Part model, mm, in its own coordinate system. Coordinates: 2 decimals unless noted, no trailing zeros.
1) Pin check, flat tips, straight feed: pin 1 Ø1.5 at (x, y) = (-3, 7.5) entering from -Z; pin 2 Ø2.5 at (x, z) = (0.5, -60) entering from +Y; pin 3 Ø1 at (y, z) = (-3, 109) entering from +X; pin 4 Ø1.6 at (y, z) = (0.5, -57.5) entering from -X. Stop position of each tip, or through.
2) Mould opens along Y. For faces 1 (the flat face through (3, 0, 152.4)), 2 (the cylindrical face through (0.782, 2.483, 2.134)) say: +Y half, -Y half, draft (parallel to the pull), parting line (faces both ways), or undercut.
3) Wall check: L1, parallel to X at y = 0, z = -15; L2, parallel to Y at x = -2, z = 47.5; L3, parallel to X at y = 3.5, z = 109.5. Give the ranges that are in metal, low to high.
```python
from build123d import *

# Parameters (mm, degrees)
SKETCH11_R              = 2.6035
FRACTIONAL_1010_1_DEPTH = 304.8


with BuildPart() as part:
    # Sketch11 → Fractional 1010(1) (new body)
    with BuildSketch(Plane.YX.offset(-152.4)):
        with BuildLine():
            Line((10.5918, 12.7), (10.5664, 12.7))
            ThreePointArc((10.5664, 12.7), (10.0584, 12.192), (9.5504, 12.7))
            Line((9.5504, 12.7), (6.3246, 12.7))
            ThreePointArc((6.3246, 12.7), (5.8166, 12.192), (5.3086, 12.7))
            Line((5.3086, 12.7), (4.3561, 12.7))
            ThreePointArc((4.3561, 12.7), (3.2512, 11.5951), (4.3561, 10.4902))
            Line((4.3561, 10.4902), (6.370083786, 10.4902))
            ThreePointArc((6.370083786, 10.4902), (7.348856743, 9.836204819), (7.119204175, 8.681663397))
            Line((7.119204175, 8.681663397), (3.88464389, 5.447103113))
            ThreePointArc((3.88464389, 5.447103113), (2.854599758, 4.758849627), (1.63957986, 4.517167143))
            Line((1.63957986, 4.517167143), (-1.63957986, 4.517167143))
            ThreePointArc((-1.63957986, 4.517167143), (-2.854599758, 4.758849627), (-3.88464389, 5.447103113))
            Line((-3.88464389, 5.447103113), (-7.119204175, 8.681663397))
            ThreePointArc((-7.119204175, 8.681663397), (-7.348856743, 9.836204819), (-6.370083786, 10.4902))
            Line((-6.370083786, 10.4902), (-4.3561, 10.4902))
            ThreePointArc((-4.3561, 10.4902), (-3.2512, 11.5951), (-4.3561, 12.7))
            Line((-4.3561, 12.7), (-5.3086, 12.7))
            ThreePointArc((-5.3086, 12.7), (-5.8166, 12.192), (-6.3246, 12.7))
            Line((-6.3246, 12.7), (-9.5504, 12.7))
            ThreePointArc((-9.5504, 12.7), (-10.0584, 12.192), (-10.5664, 12.7))
            Line((-10.5664, 12.7), (-10.5918, 12.7))
            ThreePointArc((-10.5918, 12.7), (-12.082522516, 12.082522516), (-12.7, 10.5918))
            Line((-12.7, 10.5918), (-12.7, 10.5664))
            ThreePointArc((-12.7, 10.5664), (-12.192, 10.0584), (-12.7, 9.5504))
            Line((-12.7, 9.5504), (-12.7, 6.3246))
            ThreePointArc((-12.7, 6.3246), (-12.192, 5.8166), (-12.7, 5.3086))
            Line((-12.7, 5.3086), (-12.7, 4.3561))
            ThreePointArc((-12.7, 4.3561), (-11.5951, 3.2512), (-10.4902, 4.3561))
            Line((-10.4902, 4.3561), (-10.4902, 6.370083786))
            ThreePointArc((-10.4902, 6.370083786), (-9.836204819, 7.348856743), (-8.681663397, 7.119204175))
            Line((-8.681663397, 7.119204175), (-5.447103113, 3.88464389))
            ThreePointArc((-5.447103113, 3.88464389), (-4.758849627, 2.854599758), (-4.517167143, 1.63957986))
            Line((-4.517167143, 1.63957986), (-4.517167143, -1.63957986))
            ThreePointArc((-4.517167143, -1.63957986), (-4.758849627, -2.854599758), (-5.447103113, -3.88464389))
            Line((-5.447103113, -3.88464389), (-8.681663397, -7.119204175))
            ThreePointArc((-8.681663397, -7.119204175), (-9.836204819, -7.348856743), (-10.4902, -6.370083786))
            Line((-10.4902, -6.370083786), (-10.4902, -4.3561))
            ThreePointArc((-10.4902, -4.3561), (-11.5951, -3.2512), (-12.7, -4.3561))
            Line((-12.7, -4.3561), (-12.7, -5.3086))
            ThreePointArc((-12.7, -5.3086), (-12.192, -5.8166), (-12.7, -6.3246))
            Line((-12.7, -6.3246), (-12.7, -9.5504))
            ThreePointArc((-12.7, -9.5504), (-12.192, -10.0584), (-12.7, -10.5664))
            Line((-12.7, -10.5664), (-12.7, -10.5918))
            ThreePointArc((-12.7, -10.5918), (-12.082522516, -12.082522516), (-10.5918, -12.7))
            Line((-10.5918, -12.7), (-10.5664, -12.7))
            ThreePointArc((-10.5664, -12.7), (-10.0584, -12.192), (-9.5504, -12.7))
            Line((-9.5504, -12.7), (-6.3246, -12.7))
            ThreePointArc((-6.3246, -12.7), (-5.8166, -12.192), (-5.3086, -12.7))
            Line((-5.3086, -12.7), (-4.3561, -12.7))
            ThreePointArc((-4.3561, -12.7), (-3.2512, -11.5951), (-4.3561, -10.4902))
            Line((-4.3561, -10.4902), (-6.370083786, -10.4902))
            ThreePointArc((-6.370083786, -10.4902), (-7.348856743, -9.836204819), (-7.119204175, -8.681663397))
            Line((-7.119204175, -8.681663397), (-3.88464389, -5.447103113))
            ThreePointArc((-3.88464389, -5.447103113), (-2.854599758, -4.758849627), (-1.63957986, -4.517167143))
            Line((-1.63957986, -4.517167143), (1.63957986, -4.517167143))
            ThreePointArc((1.63957986, -4.517167143), (2.854599758, -4.758849627), (3.88464389, -5.447103113))
            Line((3.88464389, -5.447103113), (7.119204175, -8.681663397))
            ThreePointArc((7.119204175, -8.681663397), (7.348856743, -9.836204819), (6.370083786, -10.4902))
            Line((6.370083786, -10.4902), (4.3561, -10.4902))
            ThreePointArc((4.3561, -10.4902), (3.2512, -11.5951), (4.3561, -12.7))
            Line((4.3561, -12.7), (5.3086, -12.7))
            ThreePointArc((5.3086, -12.7), (5.8166, -12.192), (6.3246, -12.7))
            Line((6.3246, -12.7), (9.5504, -12.7))
            ThreePointArc((9.5504, -12.7), (10.0584, -12.192), (10.5664, -12.7))
            Line((10.5664, -12.7), (10.5918, -12.7))
            ThreePointArc((10.5918, -12.7), (12.082522516, -12.082522516), (12.7, -10.5918))
            Line((12.7, -10.5918), (12.7, -10.5664))
            ThreePointArc((12.7, -10.5664), (12.192, -10.0584), (12.7, -9.5504))
            Line((12.7, -9.5504), (12.7, -6.3246))
            ThreePointArc((12.7, -6.3246), (12.192, -5.8166), (12.7, -5.3086))
            Line((12.7, -5.3086), (12.7, -4.3561))
            ThreePointArc((12.7, -4.3561), (11.5951, -3.2512), (10.4902, -4.3561))
            Line((10.4902, -4.3561), (10.4902, -6.370083786))
            ThreePointArc((10.4902, -6.370083786), (9.836204819, -7.348856743), (8.681663397, -7.119204175))
            Line((8.681663397, -7.119204175), (5.447103113, -3.88464389))
            ThreePointArc((5.447103113, -3.88464389), (4.758849627, -2.854599758), (4.517167143, -1.63957986))
            Line((4.517167143, -1.63957986), (4.517167143, 1.63957986))
            ThreePointArc((4.517167143, 1.63957986), (4.758849627, 2.854599758), (5.447103113, 3.88464389))
            Line((5.447103113, 3.88464389), (8.681663397, 7.119204175))
            ThreePointArc((8.681663397, 7.119204175), (9.836204819, 7.348856743), (10.4902, 6.370083786))
            Line((10.4902, 6.370083786), (10.4902, 4.3561))
            ThreePointArc((10.4902, 4.3561), (11.5951, 3.2512), (12.7, 4.3561))
            Line((12.7, 4.3561), (12.7, 5.3086))
            ThreePointArc((12.7, 5.3086), (12.192, 5.8166), (12.7, 6.3246))
            Line((12.7, 6.3246), (12.7, 9.5504))
            ThreePointArc((12.7, 9.5504), (12.192, 10.0584), (12.7, 10.5664))
            Line((12.7, 10.5664), (12.7, 10.5918))
            ThreePointArc((12.7, 10.5918), (12.082522516, 12.082522516), (10.5918, 12.7))
        make_face()
        Circle(SKETCH11_R, mode=Mode.SUBTRACT)
    extrude(amount=FRACTIONAL_1010_1_DEPTH)


solid = part.part
```
Geometry check:
1. pin 1: passes through
1. pin 2: stops at y = 4.52
1. pin 3: stops at x = 12.29
1. pin 4: stops at x = -4.52
2. face 1: draft
2. face 2: undercut
3. L1: x = -4.52 to -2.6, 2.6 to 4.52
3. L2: y = -4.54 to -1.67, 1.67 to 4.54
3. L3: x = -12.29 to -10.9, -5.12 to 5.12, 10.9 to 12.29
